Could you check a few things on this model? Use its own coordinates, in mm. Face numbers are marked on the shaded views. A direction names the side the tool comes from. Give positions to 0.01 mm unless a question says otherwise; leave off trailing zeros. Loops run counter-clockwise (first coordinate to the right, second up) from the corner with the lowest first, then second, coordinate; pieces in that order, holes last.
1. For P1, Ø4, axis at y = -33, z = 2, coming from the +X side; P2, Ø6, axis at y = -15, z = 6.5, coming from the -X side; P3, Ø10, axis at y = -31, z = 7, coming from the -X side, each with a flat end and sliding along its axis, tell me the tip position at first contact or that it passes through.
2. Imagine slicing it at B-B (z = 2). List the corners of the cut face in (x, y) for me.
3. Imagine slicing it at A-A (x = 5.5). List the corners of the cut face in (y, z) for me, plus the area to 3 significant figures.
4. Thinking about a two-plate mould opening in Z: for the marked faces 1, 2, 3 and 4, which applies, +Z half, -Z half, draft (parallel to the pull), parting line (faces both ways), or undercut?
5. Imagine slicing it at C-C (y = -22.5). List the corners of the cut face in (x, z) for me, plus the area to 3 significant figures.
6. For the marked faces 5, 6, 7 and 8, which set-ups out of +Z, -Z, +X, -X, +Y, -Y let a thin tool reach every point of the face, with its end or its side?
7. I need wall thicknesses on line 1 along Y through (x, z) = (-6.25, -2); line 2 along Z through (x, y) = (0, -22); line 3 along Y through (x, z) = (0.75, 8.75). Which ranges of each line are inside material? Lowest first, please.
8. Imagine slicing it at D-D (x = 1.25). List the corners of the cut face in (y, z) for me, plus the area to 3 significant figures.
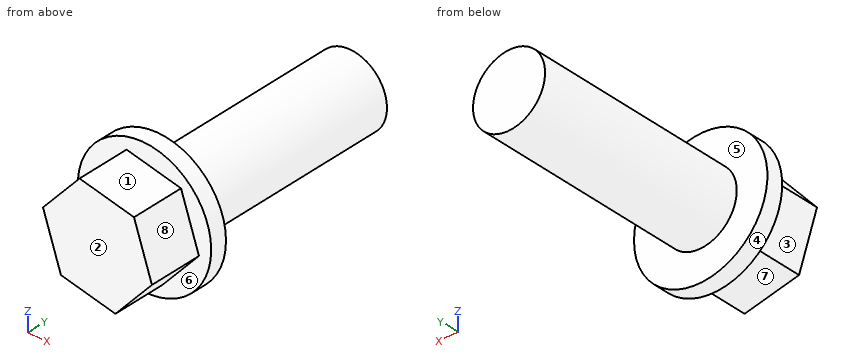
```python
from build123d import *

# Parameters (mm, degrees)
F0_R     = 5
F1_DEPTH = 29.76
F3_R     = 9.25
F4_DEPTH = 2.3
F7_DEPTH = 7.3


with BuildPart() as f1:
    # F0 (on Front) → F1 (new body)
    with BuildSketch(Plane.XZ):
        Circle(F0_R)
    extrude(amount=F1_DEPTH)

    # F3 (on offset) → F4 (join)
    with BuildSketch(Plane.XZ.offset(29.76)):
        Circle(F3_R)
    extrude(amount=F4_DEPTH)

    # F6 (on offset) → F7 (join)
    with BuildSketch(Plane.XZ.offset(32.06)):
        Polygon((7.55453, -1.489656), (5.067345, 5.797587), (-2.487185, 7.287243), (-7.55453, 1.489656), (-5.067345, -5.797587), (2.487185, -7.287243), align=None)
    extrude(amount=F7_DEPTH)


solid = f1.part
```
Derived:
1. P1: stops at x = 9.25
1. P2: stops at x = -3.57
1. P3: stops at x = -9.03
2. outline: (-9.03, -32.06) - (-7.11, -32.06) - (-7.11, -39.36) - (6.36, -39.36) - (6.36, -32.06) - (9.03, -32.06) - (9.03, -29.76) - (4.58, -29.76) - (4.58, 0) - (-4.58, 0) - (-4.58, -29.76) - (-9.03, -29.76) - close
3. outline: (-39.36, -3.84) - (-32.06, -3.84) - (-32.06, -7.44) - (-29.76, -7.44) - (-29.76, 7.44) - (-32.06, 7.44) - (-32.06, 4.53) - (-39.36, 4.53) - close
3. area: 95.3 mm2
4. face 1: +Z half
4. face 2: draft
4. face 3: -Z half
4. face 4: parting line
5. outline: circle Ø10 at (0, 0)
5. area: 78.5 mm2
6. face 5: +Y
6. face 6: -Y
6. face 7: -Z, -X, -Y
6. face 8: +Z, +X, -Y
7. line 1: y = -39.36 to -29.76
7. line 2: z = -5 to 5
7. line 3: y = -32.06 to -29.76
8. outline: (-39.36, -7.04) - (-32.06, -7.04) - (-32.06, -9.17) - (-29.76, -9.17) - (-29.76, -4.84) - (0, -4.84) - (0, 4.84) - (-29.76, 4.84) - (-29.76, 9.17) - (-32.06, 9.17) - (-32.06, 6.55) - (-39.36, 6.55) - close
8. area: 430 mm2
